Input: part model. Units: mm. Frame: model coordinates. A direction names the side the tool comes from. Round coordinates to 2 decimals unless told otherwise and drop trailing zeros. Loops run counter-clockwise (first coordinate to the right, second up) from the corner with the lowest first, then second, coordinate; pieces in that order, holes last. Notation, with made-up numbers: (-8, 23.25) - (41, 23.25) arc R23 ccw to (41, 40.25) - close; hole circle Ø1 at (83, -10.75). An arc over 180 degrees is marked (long way). Write each question's results on one line, items separated by ' | '.
from build123d import *

# Parameters (mm, degrees)
F0_W     = 10.6
F0_H     = 12.954
F1_DEPTH = 6.35
F2_W     = 8
F2_H     = 3.17
F3_DEPTH = 6.351
F4_W     = 6.35
F4_H     = 2.03
F5_DEPTH = 8.695
F6_R     = 3.17499
F9_DEPTH = 2.031


# Not quite as in the source:
# - a fillet or chamfer is up to 0.001 mm smaller than in the source, because OpenCascade refuses the exact size
# - a pattern or mirror of a feature is missing from the dataset's text; its kind, count and spacing are read off the source's solid


with BuildPart() as f1:
    # F0 (on Right) → F1 (new body)
    with BuildSketch(Plane.YZ):
        with Locations((5.3, 6.477)):
            Rectangle(F0_W, F0_H)
    extrude(amount=-F1_DEPTH)

    # F2 (on face) → F3 (cut, through all)
    with BuildSketch(Plane.YZ):
        with Locations((6.6, 6.785)):
            Rectangle(F2_W, F2_H)
    extrude(amount=-F3_DEPTH, mode=Mode.SUBTRACT)

    # F4 (on face) → F5 (join)
    with BuildSketch(Plane.YZ):
        with Locations((5.775, 1.015)):
            Rectangle(F4_W, F4_H)
    f5 = extrude(amount=F5_DEPTH)

    # F5_copies: F5 across plane
    add(f5.mirror(Plane(origin=(-3.174997, 0, 0), x_dir=(0, 0, -1), z_dir=(-1, 0, 0))))

    # F6 (radius 3.175 in the source; OpenCascade refuses exactly that, so slightly less here)
    f6_edges = [f1.edges().sort_by_distance(p)[0] for p in [
        (8.695, 2.6, 1.015),
        (8.695, 8.95, 1.015),
        (-15.044994, 8.95, 1.015),
        (-15.044994, 2.6, 1.015),
    ]]
    fillet(f6_edges, radius=F6_R)

    # F8 (on face) → F9 (cut, through all)
    with BuildSketch(Plane.XY.offset(2.03)):
        with BuildLine():
            Line((2.47, 4.15), (5.57, 4.15))
            ThreePointArc((5.57, 4.15), (7.195, 5.775), (5.57, 7.4))
            Line((5.57, 7.4), (2.47, 7.4))
            ThreePointArc((2.47, 7.4), (0.845, 5.775), (2.47, 4.15))
        make_face()
    f9 = extrude(amount=-F9_DEPTH, mode=Mode.SUBTRACT)

    # F9_copies: F9 across plane
    add(f9.mirror(Plane(origin=(-3.175, 0, 0), x_dir=(0, 0, -1), z_dir=(-1, 0, 0))), mode=Mode.SUBTRACT)


solid = f1.part
1. Section query C-C, the plane y = 8.5. Output: boundary loops of the cut face in (x, z), plus the area to 3 significant figures.
Answer:
outline: (-13.5, 0) - (7.15, 0) - (7.15, 2.03) - (0, 2.03) - (0, 5.2) - (-6.35, 5.2) - (-6.35, 2.03) - (-13.5, 2.03) - close; (-6.35, 8.37) - (0, 8.37) - (0, 12.95) - (-6.35, 12.95) - close | area: 91.2 mm^2
2. Contact query for flat-ended pins moving along their axis: pin 1 (1 mm diameter, centred on x = -10, z = 1, fed in from -Y); pin 2 (3 mm diameter, centred on x = 5, y = 1.5, fed in from +Z); pin 3 (2 mm diameter, centred on x = 2.5, z = 0.5, fed in from +Y). Output: stop coordinate, or through.
Answer:
pin 1: y = 2.6 | pin 2: z = 2.03 | pin 3: y = 8.95
3. Section query B-B, the plane y = 5.25. Output: boundary loops of the cut face in (x, z), plus the area to 3 significant figures.
Answer:
outline: (-15, 0) - (-13.46, 0) - (-13.46, 2.03) - (-15, 2.03) - close; (-7.28, 0) - (0.93, 0) - (0.93, 2.03) - (0, 2.03) - (0, 5.2) - (-6.35, 5.2) - (-6.35, 2.03) - (-7.28, 2.03) - close; (-6.35, 8.37) - (0, 8.37) - (0, 12.95) - (-6.35, 12.95) - close; (7.11, 0) - (8.65, 0) - (8.65, 2.03) - (7.11, 2.03) - close | area: 72.2 mm^2
4. Mould query, pull axis X, two halves, no side actions, for faces 6 (the flat face through (-3, 2.6, 7)), 7 (the cylindrical face through (0.845, 5.811, 1.029)), 8 (the cylindrical face through (7.79, 7.995, 1.029)). Classes: pulls with the +X half, pulls with the -X half, needs draft (parallel to the pull), parting line crosses it, or undercut.
Answer:
face 6: needs draft | face 7: undercut | face 8: pulls with the +X half
5. Line query: line 1 (X direction, y = 7, z = 1); line 2 (Y direction, x = -3, z = 5.25); line 3 (X direction, y = 3, z = 10.75). Output: solid intervals per line, ascending. Write a range as [from, to].
Answer:
line 1: [-14.8, -12.99], [-7.75, 1.4], [6.64, 8.45] | line 2: [0, 2.6] | line 3: [-6.35, 0]
6. Section query A-A, the plane x = -11.25. Output: boundary loops of the cut face in (y, z).
Answer:
outline: (2.6, 0) - (4.15, 0) - (4.15, 2.03) - (2.6, 2.03) - close; (7.4, 0) - (8.95, 0) - (8.95, 2.03) - (7.4, 2.03) - close
7. Set-up query: faces 1 (the flat face through (3, 2.6, 1)), 2 (the flat face through (-11, 4, 2.03)), 3 (the flat face through (3, 8.95, 1)), 4 (the flat face through (-10, 7.4, 1)), 5 (the flat face through (-9, 2.6, 1)). Return all of +Z, -Z, +X, -X, +Y, -Y with unobstructed straight access to the full face (end or side cutting, diameter ignored); none if empty.
Answer:
face 1: +Z, -Z, +X, -Y | face 2: +Z, -X, +Y, -Y | face 3: +Z, -Z, +X, +Y | face 4: +Z, -Z | face 5: +Z, -Z, -X, -Y
8. Section query D-D, the plane x = -5.25. Output: boundary loops of the cut face in (y, z).
Answer:
outline: (0, 0) - (10.6, 0) - (10.6, 5.2) - (2.6, 5.2) - (2.6, 8.37) - (10.6, 8.37) - (10.6, 12.95) - (0, 12.95) - close
